from build123d import *

# Parameters (mm, degrees)
SKETCH1_W           = 63.5
SKETCH1_H           = 31.75
BOSS_EXTRUDE1_DEPTH = 1
BOSS_EXTRUDE2_DEPTH = 1


with BuildPart() as part:
    # Sketch1 → Boss-Extrude1 (new body)
    with BuildSketch(Plane(origin=(0, 0, 0), x_dir=(1, 0, 0), z_dir=(0, 1, 0))):
        Rectangle(SKETCH1_W, SKETCH1_H)
    extrude(amount=BOSS_EXTRUDE1_DEPTH)

    # Sketch2 → Boss-Extrude2 (add)
    with BuildSketch(Plane(origin=(0, 0, -15.875), x_dir=(-1, 0, 0), z_dir=(0, 0, -1))):
        with BuildLine():
            Line((31.75, -17.789177687), (31.75, -43.682471344))
            Line((31.75, -43.682471344), (17.274395694, -43.682471344))
            ThreePointArc((17.274395694, -43.682471344), (15.478784489, -30.222698339), (10.02009663, -17.789177687))
            ThreePointArc((10.02009663, -17.789177687), (-2.413824992, -9.328234834), (-17.453421679, -9.350424234))
            ThreePointArc((-17.453421679, -9.350424234), (-27.026572228, -7.52456476), (-31.75, 1))
            Line((-31.75, 1), (31.75, 1))
            Line((31.75, 1), (31.75, -17.789177687))
        make_face()
        with BuildLine():
            ThreePointArc((14.682172322, -5.461834054), (19.319604518, -9.339676808), (25.284625693, -10.320474532))
            ThreePointArc((25.284625693, -10.320474532), (27.289464402, -12.805118584), (24.096851126, -12.797716819))
            ThreePointArc((24.096851126, -12.797716819), (17.34915582, -11.158394953), (12.353647921, -6.335152376))
            ThreePointArc((12.353647921, -6.335152376), (12.463721653, -3.08771562), (14.682172322, -5.461834054))
        make_face(mode=Mode.SUBTRACT)
    boss_extrude2 = extrude(amount=-BOSS_EXTRUDE2_DEPTH)

    # Mirror1: Boss-Extrude2 across plane
    add(boss_extrude2.mirror(Plane.XY))


solid = part.part
Design review of the part built by this model. Coordinates are the model's own, in mm. A direction names the side the tool comes from. Round coordinates to 2 decimals unless told otherwise and drop trailing zeros. Write each loop counter-clockwise with the first axis right and the second up, starting at its lowest first coordinate (ties: lowest second). Pieces come first, ordered by that corner, then holes. Notation, with made-up numbers: (32, -39) -> (46, -39) arc R26 ccw to (46, -12) -> close; hole circle Ø10 at (65.25, -13.75). An arc over 180 degrees is marked (long way). One line per item, written item: value. Start each with the question number.
Q1. The part is to be moulded in two halves that separate along Y. For faces 4 (the face through (-12.41, -3.11, 15.38)), 5 (the face through (0, 1, 0)), 6 (the face through (-31.75, 0.3, 0.1)), say which applies: pulls with the +Y half, pulls with the -Y half, needs draft (parallel to the pull), parting line crosses it, or undercut.
Q2. Add section B-B (y = -33). Give the boundary of the cut face in (x, z) (3 decimals).
Q3. Add section C-C (z = 6). Give the boundary of the cut face in (x, y).
Q4. To check wall thickness, follow probe 1 along Z at (x, y) = (-27.5, -9) (3 decimals); probe 2 along Y at (x, z) = (2, -8); probe 3 along X at (y, z) = (-32.5, 15). State the ranges of each line that lie inside material, in increasing order.
Q5. Tool access review of faces 1 (the face through (2.21, -9.39, 15.38)), 2 (the face through (-17.44, -11.21, 15.38)), 3 (the face through (0, 0, 0)): name each direction out of +Z, -Z, +X, -X, +Y, -Y from which nothing blocks a thin tool from reaching the whole face with its end or side.
Q6. Insertion check: P1, Ø2, axis at x = 17, z = -5.5, coming from the -Y side; P2, Ø2, axis at x = -13.08, y = -4.73, coming from the +Z side; P3, Ø5.5, axis at x = -13.08, y = -4.73, coming from the -Z side (3 decimals). Each pin has a flat end and moves straight along its axis. Give the tip position at first contact, or say it passes through.
Q7. Add section A-A (x = -13.5). Give the boundary of the cut face in (y, z) (3 decimals), then the cut area to 3 significant figures.
Q8. Add section D-D (x = 2). Give the boundary of the cut face in (y, z) (3 decimals).
Response:
1. face 4: undercut
1. face 5: pulls with the +Y half
1. face 6: needs draft
2. outline: (-31.75, -15.875) -> (-16.169, -15.875) -> (-16.169, -14.875) -> (-31.75, -14.875) -> close; (-31.75, 14.875) -> (-16.169, 14.875) -> (-16.169, 15.875) -> (-31.75, 15.875) -> close
3. outline: (-31.75, 0) -> (31.75, 0) -> (31.75, 1) -> (-31.75, 1) -> close
4. probe 1: z = -15.875 to -14.875, 14.875 to 15.875
4. probe 2: y = 0 to 1
4. probe 3: x = -31.75 to -16.06
5. face 1: +Z, -Z, -Y
5. face 2: +Z, -Z
5. face 3: +X, -X, -Y
6. P1: stops at y = 0
6. P2: passes through
6. P3: stops at z = -15.875
7. outline: (-24.543, -15.875) -> (-7.964, -15.875) -> (-7.964, -14.875) -> (-24.543, -14.875) -> close; (-24.543, 14.875) -> (-7.964, 14.875) -> (-7.964, 15.875) -> (-24.543, 15.875) -> close; (-3.026, -15.875) -> (1, -15.875) -> (1, 15.875) -> (-3.026, 15.875) -> (-3.026, 14.875) -> (0, 14.875) -> (0, -14.875) -> (-3.026, -14.875) -> close
7. area: 71.0 mm^2
8. outline: (-9.459, -15.875) -> (1, -15.875) -> (1, 15.875) -> (-9.459, 15.875) -> (-9.459, 14.875) -> (0, 14.875) -> (0, -14.875) -> (-9.459, -14.875) -> close
